Geometry: final body of the model. Coordinates: model frame, mm. A direction names the side the tool comes from. Give positions to 0.01 mm unless a question says otherwise; leave off trailing zeros. Order: outer loops, then holes, each group sorted by start corner. A loop starts at its lowest first (then second) coordinate and runs counter-clockwise, first axis right, second up. Notation, with made-up numbers: M 41.25,-4.5 L 51.25,-4.5 A12 cw 51.25,-0.5 Z; hole C -20,-31 d1. An arc over 180 degrees is marked long. Write item = value, one per line. Start each with the question number.
from build123d import *

# Parameters (mm, degrees)
BOSS_EXTRUDE1_DEPTH = 3
SKETCH2_W           = 24
SKETCH2_H           = 3
CUT_EXTRUDE1_DEPTH  = 3


with BuildPart() as part:
    # Sketch1 → Boss-Extrude1 (new body)
    with BuildSketch(Plane.XY):
        Polygon((-35, 38), (-17.5, 38), (17.5, 38), (35, 38), (35, 20.5), (38, 20.5), (38, -20.5), (35, -20.5), (35, -38), (35, -41), (17.5, -41), (17.5, -38), (-17.5, -38), (-17.5, -41), (-35, -41), (-38, -41), (-38, -38), (-38, -20.5), (-35, -20.5), (-35, 20.5), (-38, 20.5), (-38, 38), align=None)
    extrude(amount=BOSS_EXTRUDE1_DEPTH)

    # Sketch2 → Cut-Extrude1 (cut)
    with BuildSketch(Plane.XY.offset(3)):
        Rectangle(SKETCH2_W, SKETCH2_H)
    extrude(amount=-CUT_EXTRUDE1_DEPTH, mode=Mode.SUBTRACT)


solid = part.part
1) Cut plane A-A (z = 0.85). Return loops of the section in (x, y).
2) Access query for faces 1 (the flat face through (-35, 0, 1)), 2 (the flat face through (35, -31, 1)), 3 (the flat face through (0, 1.5, 2)), 4 (the flat face through (35, 29, 1)). Directions: +Z, -Z, +X, -X, +Y, -Y. A direction counts if a zero-diameter tool reaches every point of the face in a straight line with its end or side. Return the directions, or none.
3) Ray query, L1, parallel to Y at x = -4, z = 2.2; L2, parallel to X at y = 11, z = 0.75; L3, parallel to Y at x = 16.5, z = 2.5. Return the intervals inside material, ascending.
4) Cut plane B-B (x = -7.5). Return loops of the section in (y, z).
5) Cut plane C-C (y = 32.5). Return loops of the section in (x, z).
6) Pin query (flat end, axial travel): pin 1 Ø1.5 at (y, z) = (9, 1) entering from -X; pin 2 Ø0.9 at (y, z) = (29, 1) entering from +X; pin 3 Ø0.9 at (x, z) = (36, 2) entering from -Y. Return the tip coordinate at first contact, or that it passes through.
7) Draft query along Y for faces 5 (the flat face through (37, -20.5, 1)), 6 (the flat face through (-12, 0, 2)), 7 (the flat face through (17.5, -40, 1)). Return one class per face: pulls with the +Y half, pulls with the -Y half, needs draft (parallel to the pull), parting line crosses it, or undercut.
8) Cut plane D-D (x = -15.5). Return loops of the section in (y, z), plus the area to 3 significant figures.
Reply:
q1.outline = M -38,-41 L -17.5,-41 L -17.5,-38 L 17.5,-38 L 17.5,-41 L 35,-41 L 35,-20.5 L 38,-20.5 L 38,20.5 L 35,20.5 L 35,38 L -38,38 L -38,20.5 L -35,20.5 L -35,-20.5 L -38,-20.5 Z; hole M -12,-1.5 L 12,-1.5 L 12,1.5 L -12,1.5 Z
q2.face_1 = +Z, -Z, -X
q2.face_2 = +Z, -Z, +X, -Y
q2.face_3 = +Z, -Z
q2.face_4 = +Z, -Z, +X, +Y
q3.L1 = -38 to -1.5, 1.5 to 38
q3.L2 = -35 to 38
q3.L3 = -38 to 38
q4.outline = M -38,0 L -1.5,0 L -1.5,3 L -38,3 Z; M 1.5,0 L 38,0 L 38,3 L 1.5,3 Z
q5.outline = M -38,0 L 35,0 L 35,3 L -38,3 Z
q6.pin_1 = -35
q6.pin_2 = 35
q6.pin_3 = -20.5
q7.face_5 = pulls with the -Y half
q7.face_6 = undercut
q7.face_7 = needs draft
q8.outline = M -38,0 L 38,0 L 38,3 L -38,3 Z
q8.area = 228 mm²
